Verification items for the finished model (mm, model axes). Face numbers are marked on the shaded views. Coordinates: 2 decimals unless noted, no trailing zeros. Order: outer loops, then holes, each group sorted by start corner. A loop starts at its lowest first (then second) coordinate and runs counter-clockwise, first axis right, second up. Notation, with made-up numbers: M 59.5,-39.75 L 79.5,-39.75 A25 ccw 79.5,-8.75 Z; hole C 77.5,50 d5. An arc over 180 degrees is marked long. Return JSON: item names as keys, results as strings. Group by question number.
Q1. Section check C-C, the plane z = 53. Count the separate pieces of the cut face and the enclosed holes in it, then the cut area to 3 significant figures.
Q2. Section check A-A, the plane y = 0. Enter the section's corners in (x, z), then the cut area to 3 significant figures.
Q3. Go/stop test with flat-tipped pins: pin 1 Ø2 at (x, y) = (17.5, 0) entering from +Z; pin 2 Ø10 at (y, z) = (19.5, 40) entering from -X; pin 3 Ø8 at (y, z) = (-7.5, 38.5) entering from -X. Record where each tip stops, or that it passes through.
Q4. Section check B-B, the plane x = 0. Enter the section's corners in (y, z).
Q5. Section check D-D, the plane z = 21. Enter the section's corners in (x, y).
Q6. Thickness scan on probe 1 along Y at (x, z) = (0, 59); probe 2 along Y at (x, z) = (0, 14); probe 3 along Y at (x, z) = (0.5, 23) (1 decimal). Record the ranges inside material, lowest first.
Q7. Mould release check, pull along X, two halves, no side actions. Record for the marked faces 1, 2 and 3: pulls with the +X half, pulls with the -X half, needs draft (parallel to the pull), parting line crosses it, or undercut.
from build123d import *

# Parameters (mm, degrees)
SKETCH1_R           = 25
SKETCH1_R_2         = 10
BOSS_EXTRUDE1_DEPTH = 70
SKETCH3_R           = 1.65
CUT_EXTRUDE1_DEPTH  = 20
CUT_EXTRUDE2_START  = -20
SKETCH4_R           = 1.65
CUT_EXTRUDE2_DEPTH  = 20


with BuildPart() as part:
    # Sketch1 → Boss-Extrude1 (new body)
    with BuildSketch(Plane.XY):
        Circle(SKETCH1_R)
        Circle(SKETCH1_R_2, mode=Mode.SUBTRACT)
    extrude(amount=BOSS_EXTRUDE1_DEPTH)

    # Sketch3 → Cut-Extrude1 (cut)
    with BuildSketch(Plane.XY.offset(70)):
        with Locations((12.374368671, 12.374368671)):
            Circle(SKETCH3_R)
        with Locations((17.5, 0)):
            Circle(SKETCH3_R)
        with Locations((12.374368671, -12.374368671)):
            Circle(SKETCH3_R)
        with Locations((0, -17.5)):
            Circle(SKETCH3_R)
        with Locations((-12.374368671, -12.374368671)):
            Circle(SKETCH3_R)
        with Locations((-17.5, 0)):
            Circle(SKETCH3_R)
        with Locations((-12.374368671, 12.374368671)):
            Circle(SKETCH3_R)
    extrude(amount=-CUT_EXTRUDE1_DEPTH, mode=Mode.SUBTRACT)

    # Sketch4 → Cut-Extrude2 (cut)
    with BuildSketch(Plane(origin=(0, 0, 0), x_dir=(-1, 0, 0), z_dir=(0, 0, -1)).offset(CUT_EXTRUDE2_START)):
        with Locations((0, 17.5)):
            Circle(SKETCH4_R)
        with Locations(Location((12.374368671, 12.374368671, 0), (0, 0, 180))):
            Circle(SKETCH4_R)
        with Locations(Location((17.5, 0, 0), (0, 0, 180))):
            Circle(SKETCH4_R)
        with Locations(Location((12.374368671, -12.374368671, 0), (0, 0, 180))):
            Circle(SKETCH4_R)
        with Locations(Location((0, -17.5, 0), (0, 0, 180))):
            Circle(SKETCH4_R)
        with Locations(Location((-12.374368671, -12.374368671, 0), (0, 0, 180))):
            Circle(SKETCH4_R)
        with Locations(Location((-17.5, 0, 0), (0, 0, 180))):
            Circle(SKETCH4_R)
        with Locations(Location((-12.374368671, 12.374368671, 0), (0, 0, 180))):
            Circle(SKETCH4_R)
    extrude(amount=CUT_EXTRUDE2_DEPTH, mode=Mode.SUBTRACT)


solid = part.part
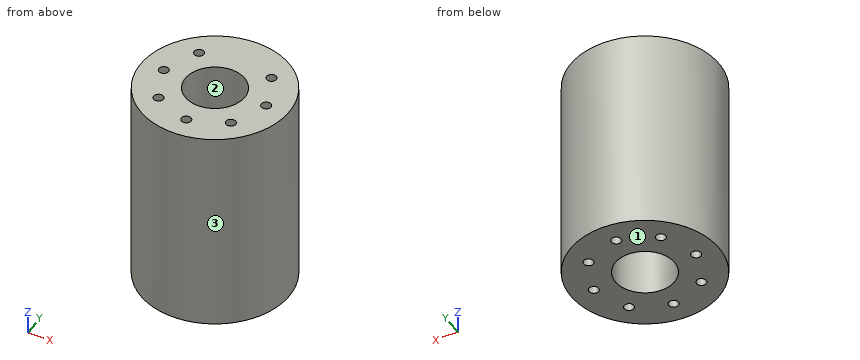
Numbers:
{
 "1": {"separate pieces": "1", "enclosed holes": "8", "area": "1,590 mm2"},
 "2": {"outline": "M -25,0 L -19.15,0 L -19.15,20 L -15.85,20 L -15.85,0 L -10,0 L -10,70 L -15.85,70 L -15.85,50 L -19.15,50 L -19.15,70 L -25,70 Z; M 10,0 L 15.85,0 L 15.85,20 L 19.15,20 L 19.15,0 L 25,0 L 25,70 L 19.15,70 L 19.15,50 L 15.85,50 L 15.85,70 L 10,70 Z", "area": "1,840 mm2"},
 "3": {"pin 1": "stops at z = 50", "pin 2": "stops at x = -20.37", "pin 3": "stops at x = -24.75"},
 "4": {"outline": "M -25,0 L -19.15,0 L -19.15,20 L -15.85,20 L -15.85,0 L -10,0 L -10,70 L -15.85,70 L -15.85,50 L -19.15,50 L -19.15,70 L -25,70 Z; M 10,0 L 15.85,0 L 15.85,20 L 19.15,20 L 19.15,0 L 25,0 L 25,70 L 10,70 Z"},
 "5": {"outline": "C 0,0 d50; hole C 0,0 d20"},
 "6": {"probe 1": "y = -25 to -19.15, -15.85 to -10, 10 to 25", "probe 2": "y = -25 to -19.15, -15.85 to -10, 10 to 15.85, 19.15 to 25", "probe 3": "y = -25 to -10, 10 to 25"},
 "7": {"face 1": "needs draft", "face 2": "undercut", "face 3": "parting line crosses it"}
}
